The listing builds one solid part. Answer for the finished solid, in the listing's coordinates (mm). A direction names the side the tool comes from. Give positions to 0.01 mm unless a question says otherwise; leave off trailing zeros. Loops run counter-clockwise (first coordinate to the right, second up) from the corner with the lowest first, then second, coordinate; pieces in that order, holes last. Notation, with made-up numbers: M 50,25 L 97,25 A26 ccw 97,40 Z; hole C -39,-20 d7. An arc over 180 degrees is marked long. One line per item, written item: value. Start each with the question number.
Q1. For faces 5 (the cylindrical face through (-3.78, 10.34, -3.7)), 6 (the flat face through (6, 0, 0)), 7 (the flat face through (-5.262, 10.057, -4.224)), determine the directions among +Z, -Z, +X, -X, +Y, -Y from which every point of the face is accessible in a straight line to the end or side of a thin tool.
Q2. Consider L1, parallel to Z at x = 0, y = 15.75; L2, parallel to Z at x = -3, y = 6.5; L3, parallel to X at y = 4, z = 0. Determine where each line is inside the solid, lowest interval first.
Q3. Flat-ended cylindrical pins translate along their axes: pin 1 (1 mm diameter, centred on x = 3.5, z = 1.5, fed in from +Y); pin 2 (1.5 mm diameter, centred on x = -2, y = 9, fed in from +Z); pin 3 (1.5 mm diameter, centred on x = -5, y = 10.5, fed in from -Z). Find the tip coordinate at first contact, or state that the pin passes through.
Q4. A cutting plane is placed at C-C, the plane z = -4.25. Determine the outline of the cut face in (x, y), and give its area (3 significant figures).
Q5. A cutting plane is placed at B-B, the plane y = 8.25. Determine the outline of the cut face in (x, z), and give its area (3 significant figures).
Q6. The mould has two halves that part along X. Classify faces 1 (the cylindrical face through (9, 10, 0)), 2 (the flat face through (-5.236, 10.057, 4.212)), 3 (the cylindrical face through (-3.78, 10.34, 3.7)), 4 (the cylindrical face through (5.097, 10.057, -0.162)): +X half, -X half, draft (parallel to the pull), parting line (faces both ways), or undercut.
Q7. A cutting plane is placed at A-A, the plane x = 0. Determine the outline of the cut face in (y, z), and give its area (3 significant figures).
Q8. A cutting plane is placed at D-D, the plane z = 0. Determine the outline of the cut face in (x, y), and give its area (3 significant figures).
from build123d import *

# Parameters (mm, degrees)
BOSS_EXTRUDE1_DEPTH = 20.4
FILLET1_R           = 1


with BuildPart() as part:
    # Sketch1 → Boss-Extrude1 (new body)
    with BuildSketch(Plane(origin=(0, 0, 0), x_dir=(1, 0, 0), z_dir=(0, 1, 0))):
        with BuildLine():
            Line((-3.709447398, -3.5), (-7.348069674, -5.196717432))
            ThreePointArc((-7.348069674, -5.196717432), (9, 0), (-7.348069674, 5.196717432))
            Line((-7.348069674, 5.196717432), (-3.709447398, 3.5))
            ThreePointArc((-3.709447398, 3.5), (5.1, 0), (-3.709447398, -3.5))
        make_face()
    extrude(amount=BOSS_EXTRUDE1_DEPTH)

    # Fillet1
    fillet1_edges = [part.edges().sort_by_distance(p)[0] for p in [
        (-3.709447398, 10.2, -3.5),
        (-7.348069674, 10.2, -5.196717432),
        (-7.348069674, 10.2, 5.196717432),
        (-3.709447398, 10.2, 3.5),
    ]]
    fillet(fillet1_edges, radius=FILLET1_R)


solid = part.part
Answer block:
1. face 5: +Y, -Y
1. face 6: +Z, -Z, +X, -X, -Y
1. face 7: -X, +Y, -Y
2. L1: -9 to -5.1, 5.1 to 9
2. L2: -8.49 to -4.12, 4.12 to 8.49
2. L3: 5.1 to 9
3. pin 1: through
3. pin 2: z = 8.91
3. pin 3: z = -7.93
4. outline: M -5.32,0 L -2.82,0 L -2.82,20.4 L -5.32,20.4 Z; M 2.82,0 L 7.93,0 L 7.93,20.4 L 2.82,20.4 Z
4. area: 155 mm^2
5. outline: M -6.47,-6.25 A9 ccw long -6.47,6.25 A1 ccw -6.18,4.65 L -4.32,3.79 A1 ccw -3.26,3.92 A5.1 cw long -3.26,-3.92 A1 ccw -4.32,-3.79 L -6.18,-4.65 A1 ccw Z
5. area: 135 mm^2
6. face 1: parting line
6. face 2: -X half
6. face 3: undercut
6. face 4: undercut
7. outline: M 0,-9 L 20.4,-9 L 20.4,-5.1 L 0,-5.1 Z; M 0,5.1 L 20.4,5.1 L 20.4,9 L 0,9 Z
7. area: 159 mm^2
8. outline: M 5.1,0 L 9,0 L 9,20.4 L 5.1,20.4 Z
8. area: 79.6 mm^2
